Verification items for the finished model (mm, model axes). Round coordinates to 2 decimals unless told otherwise and drop trailing zeros. Order: outer loops, then holes, each group sorted by start corner. A loop starts at its lowest first (then second) coordinate and runs counter-clockwise, first axis right, second up. Notation, with made-up numbers: (80, 71.5) -> (84, 71.5) arc R18 ccw to (84, 86.5) -> close; hole circle Ø5 at (-35.5, 58.25). An arc over 180 degrees is marked (long way). Answer in a Markdown table with one row per item. Add a question column.
```python
from build123d import *

# Parameters (mm, degrees)
SKETCH_1_R             = 2.5
SM_BASE_FLANGE_1_DEPTH = 3
HOLE_WIZARD_M6_1_D     = 5
HOLE_WIZARD_M6_1_DEPTH = 19
HOLE_WIZARD_M6_1_TIP   = 1.502151548


# Sheet-metal steps are written as plain solids
with BuildPart() as part:
    # Sketch 1 → 基体-法兰1 (new body)
    with BuildSketch(Plane.XY):
        Polygon((-18, 10), (18, 10), (19, 9), (19, -9), (18, -10), (-18, -10), (-19, -9), (-19, 9), align=None)
        with Locations((-14, 0)):
            Circle(SKETCH_1_R, mode=Mode.SUBTRACT)
        with Locations((14, 0)):
            Circle(SKETCH_1_R, mode=Mode.SUBTRACT)
    extrude(amount=-SM_BASE_FLANGE_1_DEPTH)

    # M6 螺纹孔1
    with Locations(Plane.XY):
        with Locations((0, 0)):
            Hole(HOLE_WIZARD_M6_1_D / 2, depth=HOLE_WIZARD_M6_1_DEPTH)
            with Locations((0, 0, -(HOLE_WIZARD_M6_1_DEPTH + HOLE_WIZARD_M6_1_TIP / 2))):  # 118° drill point
                Cone(0, HOLE_WIZARD_M6_1_D / 2, HOLE_WIZARD_M6_1_TIP, mode=Mode.SUBTRACT)


solid = part.part
```
1) Depth check by flat-ended pin: P1, Ø4, axis at x = 14, y = 0, coming from the -Z side. Enter the tip coordinate at first touch or a pass-through.
2) Draft check along Y on faces 1 (the face through (-18.5, 9.5, -1.5)), 2 (the face through (11.5, 0.1, -1.5)), 3 (the face through (-4, 0, -3)), 4 (the face through (-16.5, 0.1, -1.5)). Enter one of: +Y half, -Y half, draft (parallel to the pull), parting line (faces both ways), or undercut.
3) Cross-section at A-A, the plane y = 0. Record the boundary of the cut face in (x, z), and give its area (3 significant figures).
4) Cross-section at C-C, the plane z = -2.1. Record the boundary of the cut face in (x, y), and give its area (3 significant figures).
5) Cross-section at D-D, the plane x = 13. Record the boundary of the cut face in (y, z), and give its area (3 significant figures).
6) Thickness scan on L1, parallel to Y at x = -14, z = -1.8; L2, parallel to X at y = -2, z = -2.75; L3, parallel to Y at x = 2, z = -1. Record the ranges inside material, lowest first. Write a range as [from, to].
7) Cross-section at B-B, the plane x = -14. Record the boundary of the cut face in (y, z), and give its area (3 significant figures).
Results below:
| question | item | result |
|---|---|---|
| 1 | P1 | through |
| 2 | face 1 | +Y half |
| 2 | face 2 | undercut |
| 2 | face 3 | draft |
| 2 | face 4 | undercut |
| 3 | outline | (-19, -3) -> (-16.5, -3) -> (-16.5, 0) -> (-19, 0) -> close; (-11.5, -3) -> (-2.5, -3) -> (-2.5, 0) -> (-11.5, 0) -> close; (2.5, -3) -> (11.5, -3) -> (11.5, 0) -> (2.5, 0) -> close; (16.5, -3) -> (19, -3) -> (19, 0) -> (16.5, 0) -> close |
| 3 | area | 69.0 mm² |
| 4 | outline | (-19, -9) -> (-18, -10) -> (18, -10) -> (19, -9) -> (19, 9) -> (18, 10) -> (-18, 10) -> (-19, 9) -> close; hole circle Ø5 at (-14, 0); hole circle Ø5 at (0, 0); hole circle Ø5 at (14, 0) |
| 4 | area | 699 mm² |
| 5 | outline | (-10, -3) -> (-2.29, -3) -> (-2.29, 0) -> (-10, 0) -> close; (2.29, -3) -> (10, -3) -> (10, 0) -> (2.29, 0) -> close |
| 5 | area | 46.3 mm² |
| 6 | L1 | [-10, -2.5], [2.5, 10] |
| 6 | L2 | [-19, -15.5], [-12.5, -1.5], [1.5, 12.5], [15.5, 19] |
| 6 | L3 | [-10, -1.5], [1.5, 10] |
| 7 | outline | (-10, -3) -> (-2.5, -3) -> (-2.5, 0) -> (-10, 0) -> close; (2.5, -3) -> (10, -3) -> (10, 0) -> (2.5, 0) -> close |
| 7 | area | 45.0 mm² |
